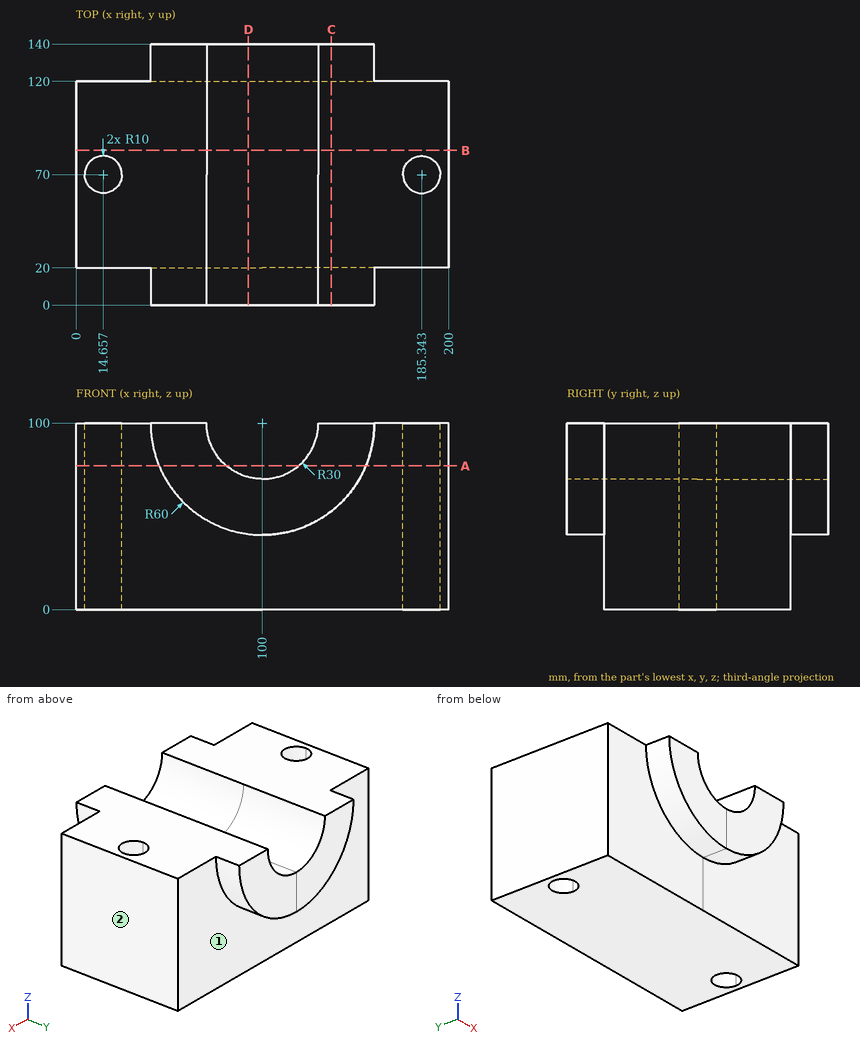
Input: dimensioned drawing with shaded views. Units: mm. Origin: part minimum x, y, z. A direction names the side the tool comes from. Give positions to 0.01 mm unless a question says otherwise; leave off trailing zeros. Write each loop counter-clockwise with the first axis right and the second up, starting at its lowest first coordinate (ties: lowest second). Pieces come first, ordered by that corner, then holes. Notation, with made-up numbers: (-18, 3) - (20, 3) arc R20 ccw to (20, 40) - close; hole circle Ø7 at (27, -37.75). An arc over 180 degrees is marked (long way). One line per item, written item: value. Start each with the question number.
Q1. Set-up query: the marked faces 1 and 2. Return all of +Z, -Z, +X, -X, +Y, -Y with unobstructed straight access to the full face (end or side cutting, diameter ignored); none if empty.
Q2. Section query B-B, the plane y = 83. Return the cut outline in (x, z), then the cut area to 3 significant figures.
Q3. Section query C-C, the plane x = 137. Return the cut outline in (y, z), then the cut area to 3 significant figures.
Q4. Material intervals for probe 1 along X at (y, z) = (65, 25); probe 2 along X at (y, z) = (64, 13); probe 3 along Y at (x, z) = (65.5, 15), sorted ascending. Write a range as from..to.
Q5. First-contact query: pin 1 Ø12 at (y, z) = (71, 48.5) entering from -X; pin 2 Ø3 at (x, y) = (83, 53) entering from +Z; pin 3 Ø8 at (x, z) = (38.5, 21.5) entering from -Y; pin 4 Ø5 at (x, y) = (91.5, 20) entering from +Z. Flat tips, straight axial feed; report the tip coordinate or a pass-through.
Q6. Section query D-D, the plane x = 92.5. Return the cut outline in (y, z), then the cut area to 3 significant figures.
Q7. Section query A-A, the plane z = 77. Return the cut outline in (x, y), then the cut area to 3 significant figures.
Answer:
1. face 1: -Z, +Y
1. face 2: +Z, -Z, +X, +Y, -Y
2. outline: (0, 0) - (200, 0) - (200, 100) - (130, 100) arc R30 cw to (70, 100) - (0, 100) - close
2. area: 18,600 mm2
3. outline: (0, 52.77) - (20, 52.77) - (20, 0) - (120, 0) - (120, 52.77) - (140, 52.77) - (140, 100) - (0, 100) - close
3. area: 11,900 mm2
4. probe 1: x = 0..6, 23.32..176.68, 194..200
4. probe 2: x = 0..6.66, 22.66..177.34, 193.34..200
4. probe 3: y = 20..120
5. pin 1: stops at x = 0
5. pin 2: stops at z = 76.38
5. pin 3: stops at y = 20
5. pin 4: stops at z = 72.09
6. outline: (0, 40.47) - (20, 40.47) - (20, 0) - (120, 0) - (120, 40.47) - (140, 40.47) - (140, 70.95) - (0, 70.95) - close
6. area: 8,310 mm2
7. outline: (0, 20) - (44.58, 20) - (44.58, 0) - (80.74, 0) - (80.74, 140) - (44.58, 140) - (44.58, 120) - (0, 120) - close; (119.26, 0) - (155.42, 0) - (155.42, 20) - (200, 20) - (200, 120) - (155.42, 120) - (155.42, 140) - (119.26, 140) - close; hole circle Ø20 at (14.66, 70); hole circle Ø20 at (185.34, 70)
7. area: 18,400 mm2
